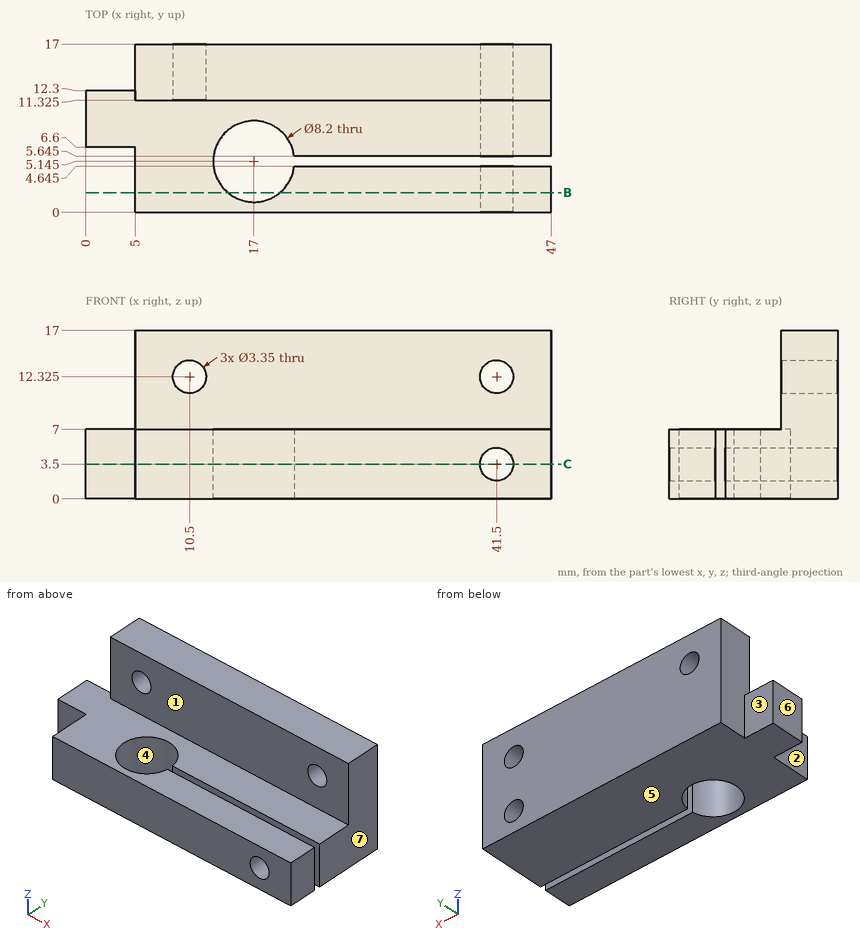
Source: three-view drawing plus pictorial views. Frame: mm from the lowest corner of the part. A direction names the side the tool comes from. Coordinates: 2 decimals unless noted, no trailing zeros. Write each loop counter-clockwise with the first axis right and the second up, starting at its lowest first coordinate (ties: lowest second). Pieces come first, ordered by that corner, then holes. Notation, with made-up numbers: (-1, 3) -> (19, 3) arc R27 cw to (19, 33) -> close; hole circle Ø3 at (81, -14.5). An arc over 180 degrees is marked (long way). Write each question's results on one line, items separated by ' | '.
Item 1: Pin query (flat end, axial travel): pin 1 Ø10 at (y, z) = (2, 2) entering from -X; pin 2 Ø10 at (x, y) = (16, 5.5) entering from +Z; pin 3 Ø6 at (y, z) = (13.5, 10) entering from -X; pin 4 Ø1.5 at (x, z) = (1.5, 4) entering from +Y. Return the tip coordinate at first contact, or that it passes through.
Conclusion:
pin 1: stops at x = 0 | pin 2: stops at z = 7 | pin 3: stops at x = 5 | pin 4: stops at y = 12.3
Item 2: Section query B-B on y = 2. Count the separate pieces of the cut face and the enclosed holes in it, plus the area to 3 significant figures.
Conclusion:
separate pieces: 2 | enclosed holes: 1 | area: 248 mm^2
Item 3: Mould query, pull axis X, two halves, no side actions, for the marked faces 4, 5, 6 and 7. Classes: +X half, -X half, draft (parallel to the pull), parting line (faces both ways), or undercut.
Conclusion:
face 4: undercut | face 5: draft | face 6: -X half | face 7: +X half
Item 4: Set-up query: the marked faces 1, 2 and 3. Return all of +Z, -Z, +X, -X, +Y, -Y with unobstructed straight access to the full face (end or side cutting, diameter ignored); none if empty.
Conclusion:
face 1: +Z, +X, -X, -Y | face 2: +Z, -Z, -X, -Y | face 3: +Z, -Z, -X, +Y
Item 5: Material intervals for probe 1 along Z at (x, y) = (10.5, 15.6); probe 2 along X at (y, z) = (3.5, 2.75) (1 decimal); probe 3 along X at (y, z) = (2, 4.75) (1 decimal), sorted ascending.
Conclusion:
probe 1: z = 0 to 10.65, 14 to 17 | probe 2: x = 5 to 13.2, 20.8 to 40, 43 to 47 | probe 3: x = 5 to 14.4, 19.6 to 40.4, 42.6 to 47
Item 6: Section query C-C on z = 3.5. Return loops of the section in (x, y) (1 decimal), plus the area to 3 significant figures.
Conclusion:
outline: (0, 6.6) -> (5, 6.6) -> (5, 0) -> (39.8, 0) -> (39.8, 4.6) -> (21.1, 4.6) arc R4.1 cw (long way) to (21.1, 5.6) -> (39.8, 5.6) -> (39.8, 17) -> (5, 17) -> (5, 12.3) -> (0, 12.3) -> close; (43.2, 0) -> (47, 0) -> (47, 4.6) -> (43.2, 4.6) -> close; (43.2, 5.6) -> (47, 5.6) -> (47, 17) -> (43.2, 17) -> close | area: 610 mm^2
